```python
from build123d import *

# Parameters (mm, degrees)
BOSS_EXTRUDE1_DEPTH = 38.1
SKETCH2_R           = 3.175
CUT_EXTRUDE1_DEPTH  = 38.1
SKETCH3_R           = 3.175
CUT_EXTRUDE2_DEPTH  = 62.234548418


with BuildPart() as part:
    # Sketch1 → Boss-Extrude1 (new body)
    with BuildSketch(Plane(origin=(0, 0, 0), x_dir=(1, 0, 0), z_dir=(0, 1, 0))):
        with BuildLine():
            Line((0, 0), (-25.4, 0))
            Line((-25.4, 0), (-25.4, 6.35))
            Line((-25.4, 6.35), (-5.120914592, 6.35))
            ThreePointArc((-5.120914592, 6.35), (10.668, 17.018), (26.456914592, 6.35))
            Line((26.456914592, 6.35), (46.736, 6.35))
            Line((46.736, 6.35), (46.736, 0))
            Line((46.736, 0), (21.336, 0))
            ThreePointArc((21.336, 0), (10.668, 10.668), (0, 0))
        make_face()
    extrude(amount=BOSS_EXTRUDE1_DEPTH)

    # Sketch2 → Cut-Extrude1 (cut)
    with BuildSketch(Plane(origin=(0, 0, -6.35), x_dir=(-1, 0, 0), z_dir=(0, 0, -1))):
        with Locations((12.7, 19.05)):
            Circle(SKETCH2_R)
    extrude(amount=-CUT_EXTRUDE1_DEPTH, mode=Mode.SUBTRACT)

    # Sketch3 → Cut-Extrude2 (cut, through all)
    with BuildSketch(Plane(origin=(0, 0, -6.35), x_dir=(-1, 0, 0), z_dir=(0, 0, -1))):
        with Locations((-34.036, 19.05)):
            Circle(SKETCH3_R)
    extrude(amount=-CUT_EXTRUDE2_DEPTH, mode=Mode.SUBTRACT)


solid = part.part
```
Check sheet for the modelled part. Datum: model origin and axes. Units: mm. A direction names the side the tool comes from. Give positions to 0.01 mm unless a question says otherwise; leave off trailing zeros. Order: outer loops, then holes, each group sorted by start corner. A loop starts at its lowest first (then second) coordinate and runs counter-clockwise, first axis right, second up. Notation, with made-up numbers: M -8.5,83 L 36.5,83 A29 cw 36.5,118 Z; hole C 70.5,-16.5 d5. An arc over 180 degrees is marked long. Answer in a Markdown table with one row per item.
1) Access from +Z, -Z, +X, -X, +Y, -Y to the whole of each face (thin tool, end or side, straight path). Record for faces 1 (the flat face through (39, 19, -6.35)), 2 (the cylindrical face through (-12.01, 15.95, -3.22)).
Filled sheet:
| item | result |
|---|---|
| face 1 | -Z, +X, +Y, -Y |
| face 2 | +Z, -Z |
2) Cross-section at C-C, the plane x = -12.7. Enter the section's corners in (y, z) (3 decimals).
Filled sheet:
| item | result |
|---|---|
| outline | M 0,-6.35 L 15.875,-6.35 L 15.875,0 L 0,0 Z; M 22.225,-6.35 L 38.1,-6.35 L 38.1,0 L 22.225,0 Z |
3) Release check for a two-part mould opening along X. For faces 3 (the cylindrical face through (10.903, 18.783, -10.665)), 4 (the cylindrical face through (34.72, 15.95, -3.22)), 5 (the flat face through (-18, 19, -6.35)), 6 (the cylindrical face through (10.385, 18.783, -17.016)) record: +X half, -X half, draft (parallel to the pull), parting line (faces both ways), or undercut.
Filled sheet:
| item | result |
|---|---|
| face 3 | undercut |
| face 4 | undercut |
| face 5 | draft |
| face 6 | parting line |
4) Cross-section at B-B, the plane z = -2.5. Enter the section's corners in (x, y) (3 decimals), plus the area to 3 significant figures.
Filled sheet:
| item | result |
|---|---|
| outline | M -25.4,0 L 0.297,0 L 0.297,38.1 L -25.4,38.1 Z; M 21.039,0 L 46.736,0 L 46.736,38.1 L 21.039,38.1 Z; hole C -12.7,19.05 d6.35; hole C 34.036,19.05 d6.35 |
| area | 1,890 mm2 |
5) Thickness scan on L1, parallel to Y at x = -12.7, z = -3.25 (3 decimals); L2, parallel to Z at x = -9, y = 9.5; L3, parallel to X at y = 24.5, z = -7.25. Record the ranges inside material, lowest first. Write a range as [from, to].
Filled sheet:
| item | result |
|---|---|
| L1 | y = [0, 15.875], [22.225, 38.1] |
| L2 | z = [-6.35, 0] |
| L3 | x = [-4.73, 2.84], [18.49, 26.06] |
6) Gauge pin test, flat ends, axial feed: P1, Ø1.5, axis at x = 23.5, y = 24.5, coming from the -Z side; P2, Ø22.5, axis at x = 39, y = 21.5, coming from the -Z side; P3, Ø5, axis at x = -3, y = 27.5, coming from the -Z side; P4, Ø10, axis at x = -12.7, y = 19.05, coming from the +Z side. Record the tip position at first contact, or that the pin passes through.
Filled sheet:
| item | result |
|---|---|
| P1 | stops at z = -11.98 |
| P2 | stops at z = -6.35 |
| P3 | stops at z = -12.84 |
| P4 | stops at z = 0 |
7) Cross-section at A-A, the plane y = 19.05. Enter the section's corners in (x, z) (3 decimals), plus the area to 3 significant figures.
Filled sheet:
| item | result |
|---|---|
| outline | M -25.4,-6.35 L -15.875,-6.35 L -15.875,0 L -25.4,0 Z; M -9.525,-6.35 L -5.121,-6.35 A17.018 ccw 26.457,-6.35 L 30.861,-6.35 L 30.861,0 L 21.336,0 A10.668 cw 0,0 L -9.525,0 Z; M 37.211,-6.35 L 46.736,-6.35 L 46.736,0 L 37.211,0 Z |
| area | 443 mm2 |
8) Cross-section at D-D, the plane y = 30. Enter the section's corners in (x, z), plus the area to 3 significant figures.
Filled sheet:
| item | result |
|---|---|
| outline | M -25.4,-6.35 L -5.12,-6.35 A17.02 ccw 26.46,-6.35 L 46.74,-6.35 L 46.74,0 L 21.34,0 A10.67 cw 0,0 L -25.4,0 Z |
| area | 523 mm2 |
